Here's how the part is built. I have some questions about the finished solid (model axes, mm). Face numbers are marked on the shaded views. A direction names the side the tool comes from. Give positions to 0.01 mm unless a question says otherwise; leave off trailing zeros. Write each loop counter-clockwise with the first axis right and the second up, starting at its lowest first coordinate (ties: lowest second). Pieces come first, ordered by that corner, then holes. Notation, with made-up numbers: (-27.75, -23.75) -> (13.25, -23.75) arc R20 cw to (13.25, 7.25) -> close; hole circle Ø8 at (4, 70). An arc over 180 degrees is marked (long way). Answer as CSV lines item,"result". Start each with the question number.
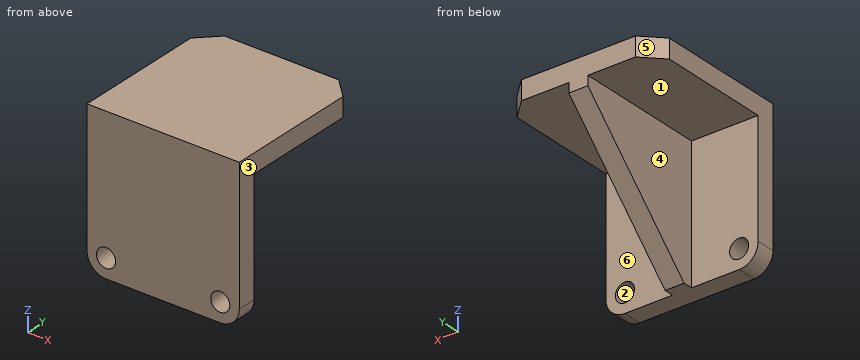
from build123d import *

# Parameters (mm, degrees)
BOSS_EXTRUDE2_DEPTH = 40
BOSS_EXTRUDE3_DEPTH = 5
FILLET1_R           = 10
SKETCH3_R           = 5
CUT_EXTRUDE1_DEPTH  = 114.578166916
CHAMFER1_SIZE       = 10


with BuildPart() as part:
    # Sketch1 → Boss-Extrude2 (new, symmetric)
    with BuildSketch(Plane(origin=(0, 0, 0), x_dir=(0, 0, -1), z_dir=(1, 0, 0))):
        Polygon((0, 0), (80, 0), (80, 10), (10, 10), (10, 80), (0, 80), align=None)
    extrude(amount=BOSS_EXTRUDE2_DEPTH, both=True)

    # Sketch2 → Boss-Extrude3 (add, symmetric)
    with BuildSketch(Plane(origin=(0, 0, 0), x_dir=(0, 0, -1), z_dir=(1, 0, 0))):
        Polygon((10, 10), (80, 10), (80, 15), (15, 80), (10, 80), align=None)
    extrude(amount=BOSS_EXTRUDE3_DEPTH, both=True)

    # Fillet1
    fillet1_edges = [part.edges().sort_by_distance(p)[0] for p in [
        (40, 5, -80),
        (-40, 5, -80),
    ]]
    fillet(fillet1_edges, radius=FILLET1_R)

    # Sketch3 → Cut-Extrude1 (cut, through all)
    with BuildSketch(Plane(origin=(0, 10, 0), x_dir=(1, 0, 0), z_dir=(0, 1, 0))):
        with Locations(Location((30, 70, 0), (0, 0, 270))):
            Circle(SKETCH3_R)
        with Locations(Location((-30, 70, 0), (0, 0, 270))):
            Circle(SKETCH3_R)
    extrude(amount=-CUT_EXTRUDE1_DEPTH, mode=Mode.SUBTRACT)

    # Chamfer1
    chamfer1_edges = [part.edges().sort_by_distance(p)[0] for p in [
        (40, 80, -5),
        (-40, 80, -5),
    ]]
    chamfer(chamfer1_edges, length=CHAMFER1_SIZE)


solid = part.part
Item 1: If we section it at A-A (y = 6.5): Please give me the cut outline in (x, z).
Item 2: For the marked faces 4, 5 and 6, which set-ups out of +Z, -Z, +X, -X, +Y, -Y let a thin tool reach every point of the face, with its end or its side?
Item 3: If we section it at D-D (x = 28): Please give me the cut outline in (y, z), and give its area (3 significant figures).
Item 4: If we section it at B-B (z = -49): Please give me the cut outline in (x, y).
Item 5: I'm going to push flat-ended pins straight in: pin 1 (3 mm diameter, centred on x = -31.5, z = -51.5, fed in from -Y); pin 2 (1 mm diameter, centred on x = -19.5, z = -23, fed in from +Y); pin 3 (3 mm diameter, centred on y = 38, z = -25.5, fed in from -X); pin 4 (17.5 mm diameter, centred on x = 31, y = 40, fed in from -Z). Where does each tip first touch, or does it pass through?
Item 6: If we section it at C-C (y = 28): Please give me the cut outline in (x, z), and give its area (3 significant figures).
Item 7: We'd pull the mould along Z, two halves only. Please class the marked faces 1, 2 and 3: released by +Z, released by -Z, zero draft, split by the parting line, or undercut.
Item 8: If I drill on line 1 (X direction, y = 6, z = -70); line 2 (X direction, y = 12, z = -26); line 3 (Z direction, x = 26, y = 37.5), over which ranges is the centre line in solid material (lowest first)? Write a range as [from, to].
Final values:
1,outline,"(-40, -70) arc R10 ccw to (-30, -80) -> (30, -80) arc R10 ccw to (40, -70) -> (40, 0) -> (-40, 0) -> close; hole circle Ø10 at (-30, -70); hole circle Ø10 at (30, -70)"
2,face 4,"-Z, -X, +Y"
2,face 5,"+Z, -Z, -X, +Y"
2,face 6,"-Z, +X, +Y"
3,outline,"(0, -80) -> (10, -80) -> (10, -74.58) -> (0, -74.58) -> close; (0, -65.42) -> (10, -65.42) -> (10, -10) -> (80, -10) -> (80, 0) -> (0, 0) -> close"
3,area,"1,410 mm2"
4,outline,"(-40, 0) -> (40, 0) -> (40, 10) -> (5, 10) -> (5, 46) -> (-5, 46) -> (-5, 10) -> (-40, 10) -> close"
5,pin 1,"y = 0"
5,pin 2,"y = 10"
5,pin 3,"x = -5"
5,pin 4,"z = -10"
6,outline,"(-40, -10) -> (-5, -10) -> (-5, -67) -> (5, -67) -> (5, -10) -> (40, -10) -> (40, 0) -> (-40, 0) -> close"
6,area,"1,370 mm2"
7,face 1,"released by -Z"
7,face 2,"undercut"
7,face 3,"zero draft"
8,line 1,"[-40, -35], [-25, 25], [35, 40]"
8,line 2,"[-5, 5]"
8,line 3,"[-10, 0]"
